The listing builds one solid part. Answer for the finished solid, in the listing's coordinates (mm). Give positions to 0.01 mm unless a question says otherwise; leave off trailing zeros. Write each loop counter-clockwise with the first axis right and the second up, starting at its lowest first coordinate (ties: lowest second). Pieces come first, ordered by that corner, then holes. Notation, with made-up numbers: (68, 87.5) - (105, 87.5) arc R8 ccw to (105, 98.5) - close; hole circle Ø4 at (-3, 34.25). An arc over 180 degrees is marked (long way). Return JSON: item names as keys, results as strings.
Autodesk Inventor part; units mm, degrees
ref_plane "YZ Plane" through (0, 0, 0) normal (1, 0, 0) x (0, 1, 0)
ref_plane "XZ Plane" through (0, 0, 0) normal (0, 1, 0) x (-1, 0, 0)
ref_plane "XY Plane" through (0, 0, 0) normal (0, 0, 1) x (1, 0, 0)
sketch "Sketch1" plane through (0, 0, 0) normal (0, 1, 0) x (-1, 0, 0)
  circle A0 centre (0, 0) radius 203.2
  line L0 (71.4375, -38.1) -> (65.0875, -38.1)
  line L1 (65.0875, -38.1) -> (65.0875, -114.3)
  line L2 (65.0875, -114.3) -> (71.4375, -114.3)
  line L3 (71.4375, -114.3) -> (71.4375, -38.1)
  line L4 (71.4375, -38.1) -> (65.0875, -114.3) construction
  line L5 (65.0875, -38.1) -> (71.4375, -114.3) construction
  line L6 (71.4375, 114.3) -> (65.0875, 114.3)
  line L7 (65.0875, 114.3) -> (65.0875, 38.1)
  line L8 (65.0875, 38.1) -> (71.4375, 38.1)
  line L9 (71.4375, 38.1) -> (71.4375, 114.3)
  line L10 (71.4375, 114.3) -> (65.0875, 38.1) construction
  line L11 (65.0875, 114.3) -> (71.4375, 38.1) construction
  line L12 (-65.0875, -38.1) -> (-71.4375, -38.1)
  line L13 (-71.4375, -38.1) -> (-71.4375, -114.3)
  line L14 (-71.4375, -114.3) -> (-65.0875, -114.3)
  line L15 (-65.0875, -114.3) -> (-65.0875, -38.1)
  line L16 (-65.0875, -38.1) -> (-71.4375, -114.3) construction
  line L17 (-71.4375, -38.1) -> (-65.0875, -114.3) construction
  line L18 (-65.0875, 114.3) -> (-71.4375, 114.3)
  line L19 (-71.4375, 114.3) -> (-71.4375, 38.1)
  line L20 (-71.4375, 38.1) -> (-65.0875, 38.1)
  line L21 (-65.0875, 38.1) -> (-65.0875, 114.3)
  line L22 (-65.0875, 114.3) -> (-71.4375, 38.1) construction
  line L23 (-71.4375, 114.3) -> (-65.0875, 38.1) construction
  line L24 (0, -284.48) -> (0, 284.48)
  line L25 (-284.48, 0) -> (284.48, 0)
  point P0 (68.2625, -76.2)
  point P1 (68.2625, 76.2)
  point P2 (-68.2625, -76.2)
  point P3 (-68.2625, 76.2)
  dimension "d0" = 406.4
  dimension "d1" = 6.35
  dimension "d2" = 6.35
  dimension "d3" = 76.2
  dimension "d4" = 6.35
  dimension "d5" = 6.35
  dimension "d6" = 76.2
  dimension "d7" = 76.2
  dimension "d8" = 76.2
  dimension "d9" = 152.4
  dimension "d10" = 152.4
extrude "Extrusion1" add sketch "Sketch1" along normal blind 6.35
properties part number "turretBasePlate"
Item 1: A cutting plane is placed at A-A on z = 70.5. Determine the outline of the cut face in (x, y).
Answer below:
{"outline": "(-190.58, 0) - (-71.44, 0) - (-71.44, 6.35) - (-190.58, 6.35) - close; (-65.09, 0) - (65.09, 0) - (65.09, 6.35) - (-65.09, 6.35) - close; (71.44, 0) - (190.58, 0) - (190.58, 6.35) - (71.44, 6.35) - close"}
Item 2: Consider L1, parallel to X at y = 2.75, z = 59.5; L2, parallel to X at y = 2.75, z = -109; L3, parallel to Z at x = 10.5, y = 3.25. Determine where each line is inside the solid, lowest interval first.
Answer below:
{"L1": "x = -194.29 to -71.44, -65.09 to 65.09, 71.44 to 194.29", "L2": "x = -171.49 to -71.44, -65.09 to 65.09, 71.44 to 171.49", "L3": "z = -202.93 to 202.93"}
Item 3: Flat-ended cylindrical pins translate along their axes: P1, Ø1.9, axis at y = 1.5, z = -69, coming from the +X side; P2, Ø3, axis at x = 139, y = 5, coming from the -Z side; P3, Ø3, axis at x = 69, y = 4, coming from the -Z side. Find the tip coordinate at first contact, or state that the pin passes through.
Answer below:
{"P1": "stops at x = 191.47", "P2": "stops at z = -149.61", "P3": "stops at z = -191.66"}
Item 4: A cutting plane is placed at D-D on x = 40. Determine the outline of the cut face in (y, z), then the cut area to 3 significant figures.
Answer below:
{"outline": "(0, -199.22) - (6.35, -199.22) - (6.35, 199.22) - (0, 199.22) - close", "area": "2,530 mm²"}
Item 5: A cutting plane is placed at C-C on z = -47. Determine the outline of the cut face in (x, y), then the cut area to 3 significant figures.
Answer below:
{"outline": "(-197.69, 0) - (-71.44, 0) - (-71.44, 6.35) - (-197.69, 6.35) - close; (-65.09, 0) - (65.09, 0) - (65.09, 6.35) - (-65.09, 6.35) - close; (71.44, 0) - (197.69, 0) - (197.69, 6.35) - (71.44, 6.35) - close", "area": "2,430 mm²"}
Item 6: A cutting plane is placed at B-B on y = 4. Determine the outline of the cut face in (x, z), then the cut area to 3 significant figures.
Answer below:
{"outline": "circle Ø406.4 at (0, 0); hole (-71.44, -114.3) - (-65.09, -114.3) - (-65.09, -38.1) - (-71.44, -38.1) - close; hole (-71.44, 38.1) - (-65.09, 38.1) - (-65.09, 114.3) - (-71.44, 114.3) - close; hole (65.09, -114.3) - (71.44, -114.3) - (71.44, -38.1) - (65.09, -38.1) - close; hole (65.09, 38.1) - (71.44, 38.1) - (71.44, 114.3) - (65.09, 114.3) - close", "area": "128,000 mm²"}
